The model under review builds one solid part; all positions refer to its coordinate system, in mm. A direction names the side the tool comes from. Coordinates: 2 decimals unless noted, no trailing zeros. Write each loop counter-clockwise with the first axis right and the second up, starting at its lowest first coordinate (ties: lowest second). Pieces come first, ordered by that corner, then holes. Notation, with made-up numbers: (-29, -22.5) -> (-15, -22.5) arc R18 ccw to (-15, -0.5) -> close; hole circle Ø10 at (74.5, 82.25). An arc over 180 degrees is marked (long way). Write each question's results on one line, items separated by ' | '.
Autodesk Fusion 360 part; units mm, degrees
sketch "Schizzo5" plane through (0, 0, 0) normal (0, 0, 1) x (1, 0, 0)
  line L0 (75.1728, 108.9816) -> (75.1728, -58.2184)
  circle A0 centre (85.1728, -55.7184) radius 1.5
  circle A1 centre (125.1728, 106.4816) radius 3
  line L1 (75.1728, 25.3816) -> (135.1728, 25.3816) construction
  circle A2 centre (85.1728, 106.4816) radius 3
  line L2 (105.1728, 25.3816) -> (122.8504, 7.7039) construction
  circle A3 centre (85.1728, 106.4816) radius 1.5
  line L3 (135.1728, 108.9816) -> (75.1728, 108.9816)
  circle A4 centre (125.1728, 106.4816) radius 1.5
  line L4 (105.1728, 25.3816) -> (87.4951, 43.0593) construction
  line L5 (105.1728, 25.3816) -> (105.1728, 1.3102) construction
  circle A5 centre (105.1728, 25.3816) radius 4.1
  line L6 (135.1728, -58.2184) -> (135.1728, 108.9816)
  line L7 (85.1728, 108.9816) -> (85.1728, -58.2184) construction
  circle A6 centre (85.1728, -55.7184) radius 3
  circle A7 centre (125.1728, -55.7184) radius 1.5
  line L8 (105.1728, 25.3816) -> (122.8504, 43.0593) construction
  line L9 (75.1728, -58.2184) -> (135.1728, -58.2184)
  circle A8 centre (125.1728, -55.7184) radius 3
  line L10 (75.1728, -55.7184) -> (135.1728, -55.7184) construction
  line L11 (105.1728, 25.3816) -> (87.4951, 7.7039) construction
  line L12 (105.1728, 108.9816) -> (105.1728, -58.2184) construction
  line L13 (105.1728, 25.3816) -> (105.1728, 56.9762) construction
  line L14 (105.1728, 25.3816) -> (105.1728, 56.9762) construction
  line L15 (105.1728, 25.3816) -> (105.1728, 1.3102) construction
  line L16 (75.1728, -45.7184) -> (135.1728, -45.7184) construction
  circle A9 centre (85.1728, -45.7184) radius 1.5
  circle A10 centre (85.1728, -45.7184) radius 3
  circle A11 centre (125.1728, -45.7184) radius 3
  circle A12 centre (125.1728, -45.7184) radius 1.5
  circle A13 centre (85.1728, 96.4816) radius 3
  circle A14 centre (85.1728, 96.4816) radius 1.5
  circle A15 centre (125.1728, 96.4816) radius 3
  circle A16 centre (125.1728, 96.4816) radius 1.5
  line L17 (107.7228, -58.2184) -> (102.6228, -58.2184)
  line L18 (102.6228, -58.2184) -> (102.6228, -53.1184)
  line L19 (102.6228, -53.1184) -> (107.7228, -53.1184)
  line L20 (107.7228, -53.1184) -> (107.7228, -58.2184)
  line L21 (107.7228, -58.2184) -> (102.6228, -53.1184) construction
  line L22 (102.6228, -58.2184) -> (107.7228, -53.1184) construction
  line L23 (102.6228, 103.8816) -> (107.7228, 103.8816)
  line L24 (102.6228, 108.9816) -> (102.6228, 103.8816)
  line L25 (107.7228, 103.8816) -> (107.7228, 108.9816)
  circle A17 centre (105.1728, 25.3816) radius 25 construction
  circle A18 centre (87.4951, 43.0593) radius 4.1
  circle A19 centre (122.8504, 7.7039) radius 4.1
  circle A20 centre (122.8504, 43.0593) radius 4.1
  circle A21 centre (87.4951, 7.7039) radius 4.1
  line L26 (87.4951, 7.7039) -> (84.596, 4.8048) construction
  line L27 (122.8504, 7.7039) -> (125.7496, 4.8048) construction
  arc A22 (84.596, 4.8048) -> (125.7496, 4.8048) centre (105.1728, 25.3816) ccw
  arc A23 (90.3942, 10.6031) -> (119.9513, 10.6031) centre (105.1728, 25.3816) ccw
  line L28 (87.4951, 43.0593) -> (84.596, 45.9584) construction
  line L29 (122.8504, 43.0593) -> (125.7496, 45.9584) construction
  arc A24 (125.7496, 45.9584) -> (84.596, 45.9584) centre (105.1728, 25.3816) ccw
  arc A25 (119.9513, 40.1601) -> (90.3942, 40.1601) centre (105.1728, 25.3816) ccw
  point P0 (105.1728, -55.6684)
  point P1 (105.1728, 25.3816)
  point P2 (87.4951, 7.7039)
  point P3 (122.8504, 7.7039)
  point P4 (122.8504, 43.0593)
  point P5 (87.4951, 43.0593)
  point P6 (84.596, 4.8048)
  point P7 (125.7496, 4.8048)
  point P8 (90.3942, 10.6031)
  point P9 (119.9513, 10.6031)
  point P10 (84.596, 45.9584)
  point P11 (125.7496, 45.9584)
  dimension "d221" = 60
  dimension "d222" = 167.2
  dimension "d223" = 2.5
  dimension "d224" = 20
  dimension "d225" = 3
  dimension "d226" = 6
  dimension "d229" = 8.2
  dimension "d350" = 3
  dimension "d351" = 6
  dimension "d354" = 10
  dimension "d355" = 5.1
  dimension "d356" = 5.1
  dimension "d361" = 50
  dimension "d362" = 8.2
  dimension "d363" = 8.2
  dimension "d364" = 45
  dimension "d365" = 45
  dimension "d366" = 45
  dimension "d367" = 45
extrude "Estrusione24" add sketch "Schizzo5" along normal blind 5 contours L0 A1 A2 L3 L6 A6 L9 A8 L18 L19 L20 L23 L24 L25
extrude "Estrusione25" add sketch "Schizzo5" along normal blind 1.8 contours A2 L3 | A6 L9 | A1 L3 | L9 A8 | A10 | A11 | A13 | A15 picked at (85.2101, 108.6469) picked at (85.2101, -57.8837) picked at (125.2101, 108.6469) picked at (125.2101, -57.8837)
sketch "Schizzo17" plane through (0, -58.2184, 0) normal (0, -1, 0) x (1, 0, 0)
  line L0 (75.1728, 0) -> (102.6228, 0)
  line L1 (102.6228, 0) -> (102.6228, 5)
  line L2 (102.6228, 5) -> (86.8311, 5)
  line L3 (86.8311, 5) -> (86.8311, 1.8)
  line L4 (86.8311, 1.8) -> (83.5144, 1.8)
  line L5 (83.5144, 1.8) -> (83.5144, 5)
  line L6 (83.5144, 5) -> (75.1728, 5)
  line L7 (75.1728, 5) -> (75.1728, 0)
  line L8 (75.1728, 5) -> (135.1728, 5) construction
  line L9 (135.1728, 5) -> (135.1728, 0) construction
  line L10 (135.1728, 0) -> (75.1728, 0) construction
  line L11 (75.1728, 0) -> (75.1728, 5) construction
  line L12 (107.7228, 0) -> (135.1728, 0) construction
  line L13 (107.7228, 5) -> (123.5144, 5) construction
  line L14 (135.1728, 0) -> (135.1728, 5) construction
  line L15 (75.1728, 2.5) -> (135.1728, 2.5) construction
  line L16 (77.9024, 5) -> (77.9024, 0) construction
  circle A0 centre (77.9024, 4.5) radius 0.4
  circle A1 centre (77.9024, 0.5) radius 0.4
  line L17 (105.1728, 5) -> (105.1728, 0) construction
  line L18 (132.4431, 5) -> (132.4431, 0) construction
  circle A2 centre (132.4431, 0.5) radius 0.4
  circle A3 centre (132.4431, 4.5) radius 0.4
  point P0 (132.4431, 4.5)
  point P1 (132.4431, 0.5)
  point P2 (132.4431, 4.5)
  dimension "d357" = 0.8
  dimension "d358" = 4
extrude "Estrusione29" cut sketch "Schizzo17" against normal blind 180 contours A0 | A1 | A2 | A3
equation "d225 = d227"
equation "d226 = d228"
equation "d350 = d227"
equation "d351 = d228"
equation "d362 = d229"
equation "d363 = d362"
Q1. Clearance check with flat-ended pins moving along their axes: P1, Ø3.5, axis at x = 85.17, y = 106.48, coming from the -Z side; P2, Ø3.5, axis at x = 125.17, y = 96.48, coming from the +Z side. State where each tip first meets the part, or that it passes through.
Solution:
P1: z = 0 | P2: z = 1.8
Q2. Add section C-C (z = 3.1). Count the separate pieces of the cut face and the enclosed holes in it, plus the area to 3 significant figures.
Solution:
separate pieces: 1 | enclosed holes: 7 | area: 8,960 mm²
Q3. Add section B-B (x = 115). Write out the cut boundary in (y, z).
Solution:
outline: (-58.22, 0) -> (-2.01, 0) -> (-2.01, 5) -> (-58.22, 5) -> close; (6.94, 0) -> (43.83, 0) -> (43.83, 5) -> (6.94, 5) -> close; (52.77, 0) -> (108.98, 0) -> (108.98, 5) -> (52.77, 5) -> close
Q4. Machinability: for faces 1 (the flat face through (135.173, 24, 2)), 2 (the flat face through (102.623, 106, 2)), 3 (the flat face through (107.723, -56, 2)), 4 (the cylindrical face through (105.403, 4.483, 2.465)), 5 (the flat face through (86, 98, 1.8)), which of the approach directions +Z, -Z, +X, -X, +Y, -Y give a long, thin tool a straight path to every point of the face, cutting with its end or side? Answer none if there is none.
Solution:
face 1: +Z, -Z, +X, +Y, -Y | face 2: +Z, -Z, +Y | face 3: +Z, -Z, -Y | face 4: +Z, -Z | face 5: +Z
Q5. Draft analysis for pull direction Y (two halves, no side actions). For faces 6 (the flat face through (105, -53.118, 2)), 7 (the cylindrical face through (88.034, 95.58, 3.378)), 8 (the flat face through (107.723, 106, 2)), state which applies: pulls with the +Y half, pulls with the -Y half, needs draft (parallel to the pull), parting line crosses it, or undercut.
Solution:
face 6: pulls with the -Y half | face 7: undercut | face 8: needs draft
Q6. For line 1 (X direction, y = -13, z = 0.4); line 2 (Y direction, x = 103.5, z = 2.35); line 3 (Y direction, x = 108.5, z = 4.6), list the stretches that pass through material, from the lowest coordinate up. Write a range as from..to.
Solution:
line 1: 75.17..77.52, 78.29..132.06, 132.83..135.17 | line 2: -53.12..-3.67, 4.55..21.64, 29.12..46.21, 54.43..103.88 | line 3: -58.22..-3.53, 4.75..22.99, 27.78..46.02, 54.29..108.98
Q7. Add section A-A (y = 8). Write out the cut boundary in (x, z).
Solution:
outline: (75.17, 0) -> (83.41, 0) -> (83.41, 5) -> (75.17, 5) -> close; (93.57, 0) -> (116.78, 0) -> (116.78, 5) -> (93.57, 5) -> close; (126.94, 0) -> (135.17, 0) -> (135.17, 5) -> (126.94, 5) -> close; hole circle Ø0.8 at (77.9, 0.5); hole circle Ø0.8 at (77.9, 4.5); hole circle Ø0.8 at (132.44, 0.5); hole circle Ø0.8 at (132.44, 4.5)
